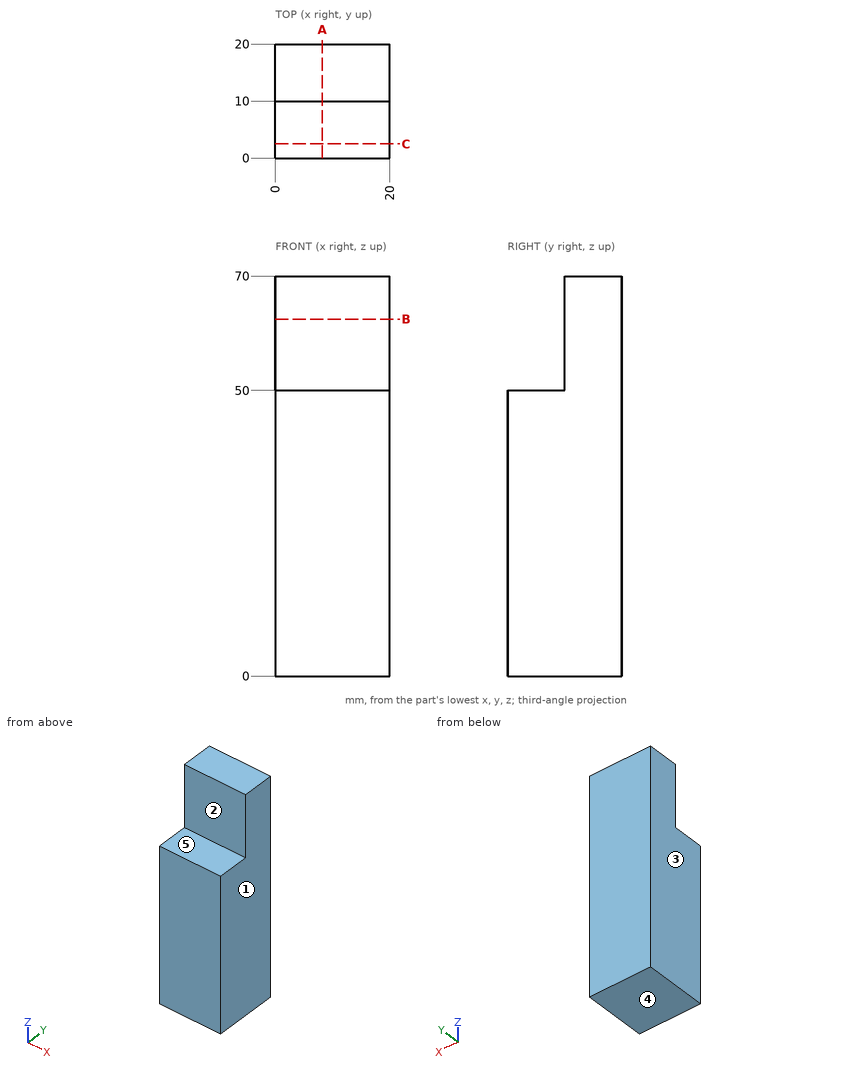
For this review, use the dimensioned drawing (mm, ordinates from the lowest corner) and the shaded views. A direction names the side the tool comes from. Round coordinates to 2 decimals unless told otherwise and drop trailing zeros. Order: outer loops, then holes, each group sorted by start corner. A loop starts at its lowest first (then second) coordinate and runs counter-clockwise, first axis right, second up. Notation, with made-up numbers: M 43.25,71 L 59.25,71 A14 cw 59.25,96 Z; hole C 19.25,46.25 d5. An arc over 180 degrees is marked long. Use a Markdown table: item, result.
1) Insertion check: pin 1 (10 mm diameter, centred on x = 3, z = 60, fed in from -Y); pin 2 (4 mm diameter, centred on x = 3, y = 4.5, fed in from +Z). Each pin has a flat end and moves straight along its axis. Give the tip position at first contact, or say it passes through.
Report:
| item | result |
|---|---|
| pin 1 | y = 10 |
| pin 2 | z = 50 |
2) Tool access review of the marked faces 4 and 5: name each direction out of +Z, -Z, +X, -X, +Y, -Y from which nothing blocks a thin tool from reaching the whole face with its end or side.
Report:
| item | result |
|---|---|
| face 4 | -Z, +X, -X, +Y, -Y |
| face 5 | +Z, +X, -X, -Y |
3) Consider section A-A (x = 8.25). Write out the cut boundary in (y, z).
Report:
| item | result |
|---|---|
| outline | M 0,0 L 20,0 L 20,70 L 10,70 L 10,50 L 0,50 Z |
4) Consider section C-C (y = 2.5). Write out the cut boundary in (x, z).
Report:
| item | result |
|---|---|
| outline | M 0,0 L 20,0 L 20,50 L 0,50 Z |
5) Consider section B-B (z = 62.5). Write out the cut boundary in (x, y), then the cut area to 3 significant figures.
Report:
| item | result |
|---|---|
| outline | M 0,10 L 20,10 L 20,20 L 0,20 Z |
| area | 200 mm^2 |
6) Wall thickness on line 1 along Z through (x, y) = (16.25, 5.5); line 2 along Y through (x, z) = (7.75, 59.5): over which ranges is each line inside the solid? List them lowest first. Write a range as [from, to].
Report:
| item | result |
|---|---|
| line 1 | [0, 50] |
| line 2 | [10, 20] |
7) Draft analysis for pull direction X (two halves, no side actions). For the marked faces 1, 2 and 3, state which applies: released by +X, released by -X, zero draft, split by the parting line, or undercut.
Report:
| item | result |
|---|---|
| face 1 | released by +X |
| face 2 | zero draft |
| face 3 | released by -X |
